Verification items for the finished model (mm, model axes). A direction names the side the tool comes from. Give positions to 0.01 mm unless a question says otherwise; leave off trailing zeros. Write each loop counter-clockwise with the first axis right and the second up, starting at its lowest first coordinate (ties: lowest second). Pieces come first, ordered by that corner, then holes. Notation, with made-up numbers: (77.25, -20.75) -> (94.25, -20.75) arc R16 ccw to (94.25, -0.75) -> close; hole circle Ø11 at (-28.5, -19). An arc over 180 degrees is marked (long way). Write item = value, one per line.
from build123d import *

# Parameters (mm, degrees)
SKETCH1_W           = 116
SKETCH1_H           = 12
BOSS_EXTRUDE1_DEPTH = 10
SKETCH2_W           = 12
SKETCH2_H           = 6
CUT_EXTRUDE1_DEPTH  = 60.160797831
SKETCH3_W           = 12
SKETCH3_H           = 6
CUT_EXTRUDE2_DEPTH  = 60.160797831
SKETCH4_RX          = 7
SKETCH4_RY          = 2.03764
CUT_EXTRUDE3_DEPTH  = 60.160797831
SKETCH5_R           = 3.000001601
CUT_EXTRUDE4_DEPTH  = 59.523499671
SKETCH6_R           = 3.000001601
CUT_EXTRUDE5_DEPTH  = 59.523499671
SKETCH7_RX          = 7
SKETCH7_RY          = 2.03764
CUT_EXTRUDE6_DEPTH  = 60.160797956


with BuildPart() as part:
    # Sketch1 → Boss-Extrude1 (new body)
    with BuildSketch(Plane.XZ.offset(5)):
        Rectangle(SKETCH1_W, SKETCH1_H)
    extrude(amount=-BOSS_EXTRUDE1_DEPTH)

    # Sketch2 → Cut-Extrude1 (cut, through all)
    with BuildSketch(Plane(origin=(0, 5, 0), x_dir=(-1, 0, 0), z_dir=(0, 1, 0))):
        with Locations((52, -3)):
            Rectangle(SKETCH2_W, SKETCH2_H)
    extrude(amount=-CUT_EXTRUDE1_DEPTH, mode=Mode.SUBTRACT)

    # Sketch3 → Cut-Extrude2 (cut, through all)
    with BuildSketch(Plane(origin=(0, 5, 0), x_dir=(-1, 0, 0), z_dir=(0, 1, 0))):
        with Locations((-52, -3)):
            Rectangle(SKETCH3_W, SKETCH3_H)
    extrude(amount=-CUT_EXTRUDE2_DEPTH, mode=Mode.SUBTRACT)

    # Sketch4 → Cut-Extrude3 (cut, through all)
    with BuildSketch(Plane.XZ.offset(5)):
        with Locations((34, 0)):
            Ellipse(SKETCH4_RX, SKETCH4_RY)
    extrude(amount=-CUT_EXTRUDE3_DEPTH, mode=Mode.SUBTRACT)

    # Sketch5 → Cut-Extrude4 (cut, through all)
    with BuildSketch(Plane(origin=(0, 0, 0), x_dir=(-1, 0, 0), z_dir=(0, 0, -1))):
        with Locations(Location((52, 0, 0), (0, 0, 90))):
            Circle(SKETCH5_R)
    extrude(amount=-CUT_EXTRUDE4_DEPTH, mode=Mode.SUBTRACT)

    # Sketch6 → Cut-Extrude5 (cut, through all)
    with BuildSketch(Plane(origin=(0, 0, 0), x_dir=(-1, 0, 0), z_dir=(0, 0, -1))):
        with Locations(Location((-52, 0, 0), (0, 0, 90))):
            Circle(SKETCH6_R)
    extrude(amount=-CUT_EXTRUDE5_DEPTH, mode=Mode.SUBTRACT)

    # Sketch7 → Cut-Extrude6 (cut, through all)
    with BuildSketch(Plane(origin=(0, 5, 0), x_dir=(-1, 0, 0), z_dir=(0, 1, 0))):
        with Locations((34, 0)):
            Ellipse(SKETCH7_RX, SKETCH7_RY)
    extrude(amount=-CUT_EXTRUDE6_DEPTH, mode=Mode.SUBTRACT)


solid = part.part
Item 1: Sectioned sample at B-B on y = 0. Give the number of separate pieces and of enclosed holes in the cut face, then the cut area to 3 significant figures.
Response values:
separate_pieces = 3
enclosed_holes = 2
area = 1,090 mm^2
Item 2: Sectioned sample at A-A on x = -52. Record the cut outline in (y, z).
Response values:
outline = (-5, 0) -> (-3, 0) -> (-3, 6) -> (-5, 6) -> close; (3, 0) -> (5, 0) -> (5, 6) -> (3, 6) -> close
Item 3: Material ranges on line 1 (X direction, y = 0, z = 3); line 2 (X direction, y = -2, z = 3.75); line 3 (X direction, y = 1.5, z = -3.5), recorded low to high.
Response values:
line_1 = -58 to -55, -49 to 49, 55 to 58
line_2 = -58 to -54.24, -49.76 to 49.76, 54.24 to 58
line_3 = -46 to 46
Item 4: Sectioned sample at C-C on x = 47.5. Record the cut outline in (y, z).
Response values:
outline = (-5, 0) -> (5, 0) -> (5, 6) -> (-5, 6) -> close
Item 5: Mould release check, pull along Y, two halves, no side actions. Record for faces 1 (the flat face through (-1, 5, 0)), 2 (the cylindrical face through (-49, 0, 3)), 3 (the flat face through (46, 0, -3)): +Y half, -Y half, draft (parallel to the pull), parting line (faces both ways), or undercut.
Response values:
face_1 = +Y half
face_2 = undercut
face_3 = draft
Item 6: Go/stop test with flat-tipped pins: P1, Ø1.5, axis at y = -3.5, z = -4.5, coming from the +X side; P2, Ø5, axis at y = -2, z = -3.5, coming from the -X side; P3, Ø3, axis at x = -50, y = -1, coming from the -Z side. Record where each tip stops, or that it passes through.
Response values:
P1 = 46
P2 = -46
P3 = 0
Item 7: Set-up check for faces 4 (the flat face through (-46, 0, -3)), 5 (the flat face through (-1, -5, 0)), 6 (the flat face through (52.1, 3.4, 0)): record each of +Z, -Z, +X, -X, +Y, -Y from which the full face is reachable in a straight line by a thin tool's end or side.
Response values:
face_4 = -Z, -X, +Y, -Y
face_5 = +Z, -Z, +X, -X, -Y
face_6 = -Z, +X, +Y, -Y
